from build123d import *

# Parameters (mm, degrees)
F0_R     = 1.7272
F1_DEPTH = 12.7
F2_R     = 1.7272
F2_R_2   = 38.1
F2_R_3   = 2.15265
F3_DEPTH = 12.7
F4_R     = 1.7272
F4_R_2   = 2.15265
F5_DEPTH = 12.7
F6_R     = 3.96875
F7_DEPTH = 6.35
F8_R     = 3.96875


# Not quite as in the source:
# - a feature names something its author has since deleted; it is built from what else it names


with BuildPart() as f1:
    # F0 (on Top) → F1 (new body)
    with BuildSketch(Plane.XY):
        Polygon((0, -177.8), (0, 0), (0, 177.8), (-1524, 177.8), (-1524, -177.8), align=None)
        with Locations((-1494.63125, -72.23125)):
            Circle(F0_R, mode=Mode.SUBTRACT)
        with Locations((-1350.16875, -72.23125)):
            Circle(F0_R, mode=Mode.SUBTRACT)
        with Locations((-1494.63125, 72.23125)):
            Circle(F0_R, mode=Mode.SUBTRACT)
        with Locations((-1350.16875, 72.23125)):
            Circle(F0_R, mode=Mode.SUBTRACT)
    extrude(amount=F1_DEPTH)

    # F2 (on face) → F3 (cut, through all)
    with BuildSketch(Plane.XY.offset(12.7)):
        with Locations((-1270.635, 0)):
            Circle(F2_R)
        with Locations((-762, -75.565)):
            Circle(F2_R)
        with Locations((-762, 75.565)):
            Circle(F2_R)
        with Locations((-253.365, 0)):
            Circle(F2_R)
        with Locations((-100.1617631794, 73.9775)):
            Circle(F2_R_2)
        with Locations((-100.1617631794, -73.9775)):
            Circle(F2_R_2)
        with Locations((-1270.635, 73.9775)):
            Circle(F2_R_2)
        with Locations((-1270.635, -73.9775)):
            Circle(F2_R_2)
        with Locations((-150.7879570619, -124.6036938825)):
            Circle(F2_R_3)
        with Locations((-49.5355692968, -124.6036938825)):
            Circle(F2_R_3)
        with Locations((-49.5355692968, -23.3513061175)):
            Circle(F2_R_3)
        with Locations((-150.7879570619, -23.3513061175)):
            Circle(F2_R_3)
        with Locations((-147.1272202412, 23.3513061175)):
            Circle(F2_R_3)
        with Locations((-147.1272202412, 124.6036938825)):
            Circle(F2_R_3)
        with Locations((-53.1963061175, 124.6036938825)):
            Circle(F2_R_3)
        with Locations((-53.1963061175, 23.3513061175)):
            Circle(F2_R_3)
        with Locations((-1321.2611938825, -124.6036938825)):
            Circle(F2_R_3)
        with Locations((-1220.0088061175, -124.6036938825)):
            Circle(F2_R_3)
        with Locations((-1220.0088061175, -23.3513061175)):
            Circle(F2_R_3)
        with Locations((-1321.2611938825, -23.3513061175)):
            Circle(F2_R_3)
        with Locations((-1321.2611938825, 23.3513061175)):
            Circle(F2_R_3)
        with Locations((-1220.0088061175, 23.3513061175)):
            Circle(F2_R_3)
        with Locations((-1220.0088061175, 124.6036938825)):
            Circle(F2_R_3)
        with Locations((-1321.2611938825, 124.6036938825)):
            Circle(F2_R_3)
    extrude(amount=-F3_DEPTH, mode=Mode.SUBTRACT)

    # F4 (on face) → F5 (cut, through all)
    with BuildSketch(Plane.XY.offset(12.7)):
        with Locations((-467.2984367897, -19.05)):
            Circle(F4_R)
        with Locations((-518.0984367897, -19.05)):
            Circle(F4_R)
        with Locations((-518.0984367897, 19.05)):
            Circle(F4_R)
        with Locations((-467.2984367897, 19.05)):
            Circle(F4_R)
        with Locations((-873.6984367897, 19.05)):
            Circle(F4_R)
        with Locations((-873.6984367897, -19.05)):
            Circle(F4_R)
        with Locations((-924.4984367897, -19.05)):
            Circle(F4_R)
        with Locations((-924.4984367897, 19.05)):
            Circle(F4_R)
        with Locations((-172.5517631794, 118.3676195)):
            Circle(F4_R_2)
        with Locations((-242.2869805794, 118.3676195)):
            Circle(F4_R_2)
        with Locations((-242.2869805794, -118.3676195)):
            Circle(F4_R_2)
        with Locations((-172.5517631794, -118.3676195)):
            Circle(F4_R_2)
        with Locations((-1198.245, -118.3676195)):
            Circle(F4_R_2)
        with Locations((-1149.509893, -118.3676195)):
            Circle(F4_R_2)
        with Locations((-1198.245, 118.3676195)):
            Circle(F4_R_2)
        with Locations((-1149.509893, 118.3676195)):
            Circle(F4_R_2)
    extrude(amount=-F5_DEPTH, mode=Mode.SUBTRACT)

    # F6 (on face) → F7 (cut)
    with BuildSketch(Plane(origin=(0, 0, 0), x_dir=(1, 0, 0), z_dir=(0, 0, -1))):
        with Locations((-924.4984367897, -19.05)):
            Circle(F6_R)
        with Locations((-873.6984367897, -19.05)):
            Circle(F6_R)
        with Locations((-873.6984367897, 19.05)):
            Circle(F6_R)
        with Locations((-924.4984367897, 19.05)):
            Circle(F6_R)
        with Locations((-467.2984367897, -19.05)):
            Circle(F6_R)
        with Locations((-467.2984367897, 19.05)):
            Circle(F6_R)
        with Locations((-518.0984367897, 19.05)):
            Circle(F6_R)
        with Locations((-518.0984367897, -19.05)):
            Circle(F6_R)
    extrude(amount=-F7_DEPTH, mode=Mode.SUBTRACT)

    # F8
    f8_edges = [f1.edges().sort_by_distance(p)[0] for p in [
        (-1524, 177.8, 6.35),
        (-1524, -177.8, 6.35),
        (0, -177.8, 6.35),
        (0, 177.8, 6.35),
    ]]
    fillet(f8_edges, radius=F8_R)


solid = f1.part
The listing builds one solid part. Answer for the finished solid, in the listing's coordinates (mm). Round coordinates to 2 decimals unless told otherwise and drop trailing zeros. Use a Markdown table: item, result. Add a question column.
1. For a pull along Y with two mould halves and no side action, classify faces 1 (the face through (-128.24, 99.73, 6.44)), 2 (the face through (-773, 2, 0)) as +Y half, -Y half, draft (parallel to the pull), parting line (faces both ways), or undercut.
2. Consider line 1 (X direction, y = 69.5, z = 5.25); line 2 (X direction, y = 19.05, z = 2); line 3 (X direction, y = 17.5, z = 4.25). Determine where each line is inside the solid, lowest interval first.
3. A flat-ended cylindrical pin translates along its axis: P1, Ø7, axis at x = -518.1, y = -19.05, coming from the -Z side. Find the tip coordinate at first contact, or state that the pin passes through.
4. The part is cut by section A-A (z = 3.75). Give the number of separate pieces and of enclosed holes in the cut face, and give its area (3 significant figures).
Reported:
| question | item | result |
|---|---|---|
| 1 | face 1 | undercut |
| 1 | face 2 | draft |
| 2 | line 1 | -1524 to -1308.47, -1232.8 to -138, -62.33 to 0 |
| 2 | line 2 | -1524 to -928.47, -920.53 to -877.67, -869.73 to -522.07, -514.13 to -471.27, -463.33 to 0 |
| 2 | line 3 | -1524 to -928.15, -920.84 to -877.35, -870.04 to -521.75, -514.44 to -470.95, -463.64 to 0 |
| 3 | P1 | z = 6.35 |
| 4 | separate pieces | 1 |
| 4 | enclosed holes | 44 |
| 4 | area | 523,000 mm^2 |
